```python
from build123d import *

# Parameters (mm, degrees)
SKETCH1_W           = 102
SKETCH1_H           = 52
SKETCH1_W_2         = 63
SKETCH1_H_2         = 8
BOSS_EXTRUDE1_DEPTH = 3
BOSS_EXTRUDE2_DEPTH = 82
SKETCH3_W           = 2
SKETCH3_H           = 48
BOSS_EXTRUDE3_DEPTH = 12
CUT_EXTRUDE1_REACH  = 144.594
SKETCH4_R           = 1.6
SKETCH5_W           = 10
SKETCH5_H           = 10
SKETCH5_W_2         = 5
SKETCH5_W_3         = 4
CUT_EXTRUDE2_DEPTH  = 1
SKETCH6_W           = 10
SKETCH6_H           = 10
SKETCH6_R           = 1.6
BOSS_EXTRUDE4_DEPTH = 4.5
CUT_EXTRUDE3_DEPTH  = 3
SKETCH8_R           = 1.75
CUT_EXTRUDE4_DEPTH  = 3
SKETCH9_R           = 1.75
CUT_EXTRUDE5_DEPTH  = 3


with BuildPart() as part:
    # Sketch1 → Boss-Extrude1 (new body)
    with BuildSketch(Plane(origin=(0, 0, 0), x_dir=(1, 0, 0), z_dir=(0, 1, 0))):
        with Locations((51, 26)):
            Rectangle(SKETCH1_W, SKETCH1_H)
        with Locations((55.5, -4)):
            Rectangle(SKETCH1_W_2, SKETCH1_H_2)
    extrude(amount=BOSS_EXTRUDE1_DEPTH)

    # Sketch2 → Boss-Extrude2 (add)
    with BuildSketch(Plane(origin=(0, 3, 0), x_dir=(1, 0, 0), z_dir=(0, 1, 0))):
        Polygon((0, 0), (0, 52), (102, 52), (102, 48), (100, 48), (100, 50), (2, 50), (2, 0), align=None)
    extrude(amount=BOSS_EXTRUDE2_DEPTH)

    # Sketch3 → Boss-Extrude3 (add)
    with BuildSketch(Plane(origin=(0, 3, 0), x_dir=(1, 0, 0), z_dir=(0, 1, 0))):
        with Locations((101, 24)):
            Rectangle(SKETCH3_W, SKETCH3_H)
    extrude(amount=BOSS_EXTRUDE3_DEPTH)

    # Sketch4 → Cut-Extrude1 (cut, up to next)
    with BuildSketch(Plane(origin=(102, 0, 0), x_dir=(0, 0, -1), z_dir=(1, 0, 0)), mode=Mode.PRIVATE) as cut_extrude1_sk1:
        with Locations((7, 7)):
            Circle(SKETCH4_R)
    cut_extrude1_tool1 = extrude(cut_extrude1_sk1.sketch, amount=-CUT_EXTRUDE1_REACH, mode=Mode.PRIVATE) & part.part
    add(cut_extrude1_tool1.solids().sort_by_distance((102, 7, -7))[0], mode=Mode.SUBTRACT)

    # Sketch5 → Cut-Extrude2 (cut)
    with BuildSketch(Plane(origin=(0, 3, 0), x_dir=(1, 0, 0), z_dir=(0, 1, 0))):
        with Locations((87, 7)):
            Rectangle(SKETCH5_W, SKETCH5_H)
        with Locations((75, 7)):
            Rectangle(SKETCH5_W, SKETCH5_H)
        with Locations((63, 7)):
            Rectangle(SKETCH5_W, SKETCH5_H)
        with Locations((51, 7)):
            Rectangle(SKETCH5_W, SKETCH5_H)
        with Locations((39, 7)):
            Rectangle(SKETCH5_W, SKETCH5_H)
        with Locations((27, 7)):
            Rectangle(SKETCH5_W, SKETCH5_H)
        with Locations((15, 7)):
            Rectangle(SKETCH5_W, SKETCH5_H)
        with Locations((75, 19)):
            Rectangle(SKETCH5_W, SKETCH5_H)
        with Locations((63, 19)):
            Rectangle(SKETCH5_W, SKETCH5_H)
        with Locations((51, 19)):
            Rectangle(SKETCH5_W, SKETCH5_H)
        with Locations((39, 19)):
            Rectangle(SKETCH5_W, SKETCH5_H)
        with Locations((27, 19)):
            Rectangle(SKETCH5_W, SKETCH5_H)
        with Locations((15, 19)):
            Rectangle(SKETCH5_W, SKETCH5_H)
        with Locations((75, 31)):
            Rectangle(SKETCH5_W, SKETCH5_H)
        with Locations((63, 31)):
            Rectangle(SKETCH5_W, SKETCH5_H)
        with Locations((51, 31)):
            Rectangle(SKETCH5_W, SKETCH5_H)
        with Locations((39, 31)):
            Rectangle(SKETCH5_W, SKETCH5_H)
        with Locations((27, 31)):
            Rectangle(SKETCH5_W, SKETCH5_H)
        with Locations((15, 31)):
            Rectangle(SKETCH5_W, SKETCH5_H)
        with Locations((75, 43)):
            Rectangle(SKETCH5_W, SKETCH5_H)
        with Locations((63, 43)):
            Rectangle(SKETCH5_W, SKETCH5_H)
        with Locations((51, 43)):
            Rectangle(SKETCH5_W, SKETCH5_H)
        with Locations((39, 43)):
            Rectangle(SKETCH5_W, SKETCH5_H)
        with Locations((27, 43)):
            Rectangle(SKETCH5_W, SKETCH5_H)
        with Locations((15, 43)):
            Rectangle(SKETCH5_W, SKETCH5_H)
        with Locations((87, 19)):
            Rectangle(SKETCH5_W, SKETCH5_H)
        with Locations((87, 31)):
            Rectangle(SKETCH5_W, SKETCH5_H)
        with Locations((87, 43)):
            Rectangle(SKETCH5_W, SKETCH5_H)
        with Locations((5.5, 7)):
            Rectangle(SKETCH5_W_2, SKETCH5_H)
        with Locations((5.5, 19)):
            Rectangle(SKETCH5_W_2, SKETCH5_H)
        with Locations((5.5, 31)):
            Rectangle(SKETCH5_W_2, SKETCH5_H)
        with Locations((5.5, 43)):
            Rectangle(SKETCH5_W_2, SKETCH5_H)
        with Locations((96, 43)):
            Rectangle(SKETCH5_W_3, SKETCH5_H)
        with Locations((96, 31)):
            Rectangle(SKETCH5_W_3, SKETCH5_H)
        with Locations((96, 19)):
            Rectangle(SKETCH5_W_3, SKETCH5_H)
        with Locations((96, 7)):
            Rectangle(SKETCH5_W_3, SKETCH5_H)
    extrude(amount=-CUT_EXTRUDE2_DEPTH, mode=Mode.SUBTRACT)

    # Sketch6 → Boss-Extrude4 (add)
    with BuildSketch(Plane(origin=(102, 0, 0), x_dir=(0, 0, -1), z_dir=(1, 0, 0))):
        with Locations((7, 7)):
            Rectangle(SKETCH6_W, SKETCH6_H)
        with Locations((7, 7)):
            Circle(SKETCH6_R, mode=Mode.SUBTRACT)
    extrude(amount=-BOSS_EXTRUDE4_DEPTH)

    # Sketch7 → Cut-Extrude3 (cut)
    with BuildSketch(Plane.ZY.offset(-97.5)):
        Polygon((-4.250369343, 8.5875), (-7, 10.175), (-9.749630657, 8.5875), (-9.749630657, 5.4125), (-7, 3.825), (-4.250369343, 5.4125), align=None)
    extrude(amount=-CUT_EXTRUDE3_DEPTH, mode=Mode.SUBTRACT)

    # Sketch8 → Cut-Extrude4 (cut)
    with BuildSketch(Plane(origin=(0, 0, -52), x_dir=(-1, 0, 0), z_dir=(0, 0, -1))):
        with Locations((-35, 49.5)):
            Circle(SKETCH8_R)
        with Locations((-35, 9.5)):
            Circle(SKETCH8_R)
        Polygon((-16.5, 14.5), (-60, 14.5), (-60, 44.5), (-16.5, 44.5), (-10, 38), (-10, 21), align=None)
    extrude(amount=-CUT_EXTRUDE4_DEPTH, mode=Mode.SUBTRACT)

    # Sketch9 → Cut-Extrude5 (cut)
    with BuildSketch(Plane.ZY):
        with Locations((-24, 67)):
            Circle(SKETCH9_R)
        with Locations((-35, 67)):
            Circle(SKETCH9_R)
    extrude(amount=-CUT_EXTRUDE5_DEPTH, mode=Mode.SUBTRACT)


solid = part.part
```
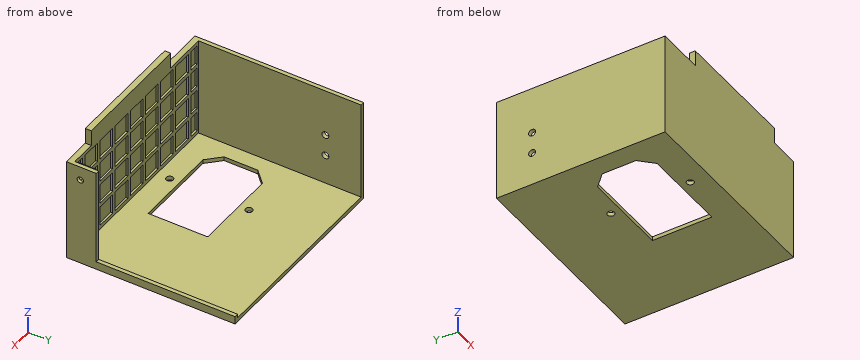
Verification items for the finished model (mm, model axes). Coordinates: 2 decimals unless noted, no trailing zeros. Loops run counter-clockwise (first coordinate to the right, second up) from the corner with the lowest first, then second, coordinate; pieces in that order, holes last. Notation, with made-up numbers: (-9, 78) -> (33, 78) arc R19 ccw to (33, 88) -> close; hole circle Ø6 at (-39.75, 27.25). An arc over 180 degrees is marked (long way). Answer in a Markdown table with one row per item. Add a question column.
1. Depth check by flat-ended pin: P1, Ø12, axis at x = 58.5, y = 76, coming from the +Z side; P2, Ø0.5, axis at x = 88.5, y = 2.5, coming from the +Z side; P3, Ø2, axis at y = 22, z = -16.5, coming from the +X side. Enter the tip coordinate at first touch or a pass-through.
2. Material ranges on probe 1 along Y at (x, z) = (35, -50.7); probe 2 along Y at (x, z) = (1.1, -24); probe 3 along X at (y, z) = (79, -48.5), recorded low to high. Write a range as [from, to].
3. Section check A-A, the plane y = 19. Enter the section's corners in (x, z), then the cut area to 3 significant figures.
4. Section check B-B, the plane x = 84. Enter the section's corners in (y, z).
5. Section check C-C, the plane y = 60.5. Enter the section's corners in (x, z).
Derived:
| question | item | result |
|---|---|---|
| 1 | P1 | stops at z = -50 |
| 1 | P2 | stops at z = 0 |
| 1 | P3 | stops at x = 2 |
| 2 | probe 1 | y = [0, 7.75], [11.25, 14.5], [44.5, 47.75], [51.25, 85] |
| 2 | probe 2 | y = [0, 65.25], [68.75, 85] |
| 2 | probe 3 | x = [0, 2], [100, 102] |
| 3 | outline | (0, -52) -> (12, -52) -> (12, -50) -> (2, -50) -> (2, 0) -> (0, 0) -> close; (60, -52) -> (102, -52) -> (102, -48) -> (100, -48) -> (100, -50) -> (60, -50) -> close |
| 3 | area | 212 mm² |
| 4 | outline | (0, -52) -> (85, -52) -> (85, -50) -> (3, -50) -> (3, -48) -> (2, -48) -> (2, -38) -> (3, -38) -> (3, -36) -> (2, -36) -> (2, -26) -> (3, -26) -> (3, -24) -> (2, -24) -> (2, -14) -> (3, -14) -> (3, -12) -> (2, -12) -> (2, -2) -> (3, -2) -> (3, 8) -> (0, 8) -> close |
| 5 | outline | (0, -52) -> (102, -52) -> (102, -48) -> (100, -48) -> (100, -50) -> (2, -50) -> (2, 0) -> (0, 0) -> close |
